Read the model definition and answer for the solid it produces. Units are mm, in the model's axes. Face numbers are marked on the shaded views. Give positions to 0.01 mm unless a question says otherwise; leave off trailing zeros. Loops run counter-clockwise (first coordinate to the right, second up) from the corner with the lowest first, then second, coordinate; pieces in that order, holes last. Notation, with made-up numbers: (75.25, -5) -> (121.25, -5) arc R26 cw to (121.25, 13) -> close; hole circle Ø1 at (-13.75, -5.75). An arc over 180 degrees is marked (long way). Answer as CSV lines item,"result". Start each with the question number.
```python
from build123d import *

# Parameters (mm, degrees)
SKETCH1_R           = 2.5
SKETCH1_R_2         = 4.9
BOSS_EXTRUDE1_DEPTH = 2


with BuildPart() as part:
    # Sketch1 → Boss-Extrude1 (new body)
    with BuildSketch(Plane.XY):
        with BuildLine():
            Line((-15, 8), (-39.191835885, 8))
            ThreePointArc((-39.191835885, 8), (0, 40), (39.191835885, 8))
            Line((39.191835885, 8), (15, 8))
            Line((15, 8), (15, -8))
            Line((15, -8), (39.191835885, -8))
            ThreePointArc((39.191835885, -8), (0, -40), (-39.191835885, -8))
            Line((-39.191835885, -8), (-15, -8))
            Line((-15, -8), (-15, 8))
        make_face()
        with Locations((0, 19.908720325)):
            Circle(SKETCH1_R, mode=Mode.SUBTRACT)
        with Locations((0, -20.091279675)):
            Circle(SKETCH1_R, mode=Mode.SUBTRACT)
        Circle(SKETCH1_R_2, mode=Mode.SUBTRACT)
    extrude(amount=BOSS_EXTRUDE1_DEPTH)


solid = part.part
```
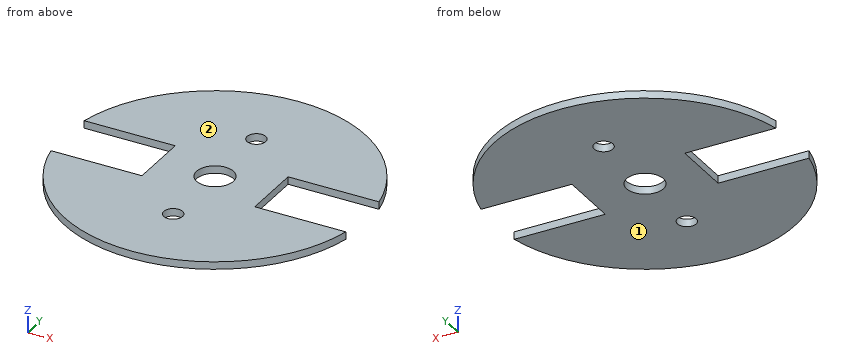
(1) Find the intervals of material crossed by line 1 along Y through (x, z) = (-1, 0.9); line 2 along X through (y, z) = (-20, 0.95); line 3 along X through (y, z) = (-2.5, 1), in increasing order. Write a range as from..to.
(2) Find section D-D on x = 0. Write down the section's boundary in (y, z), then the cut area to 3 significant figures.
(3) Find section C-C on z = 0.9. Write down the section's boundary in (x, y).
(4) Find section B-B on x = 25. Write down the section's boundary in (y, z).
(5) Each of these flat-tipped pins is pushed along its axis until it touches: P1, Ø0.6, axis at x = -28, z = 1, coming from the +Y side; P2, Ø0.6, axis at x = 22.5, z = 1, coming from the +Y side; P3, Ø1, axis at x = -29, z = 1.5, coming from the -Y side. Where does it stop, or does it pass through?
(6) Find section A-A on y = 0. Write down the section's boundary in (x, z), then the cut area to 3 significant figures.
(7) The mould has two halves that part along Z. Classify the marked faces 1 and 2: pulls with the +Z half, pulls with the -Z half, needs draft (parallel to the pull), parting line crosses it, or undercut.
Answer block:
1,line 1,"y = -39.99..-22.38, -17.8..-4.8, 4.8..17.62, 22.2..39.99"
1,line 2,"x = -34.64..-2.5, 2.5..34.64"
1,line 3,"x = -15..-4.21, 4.21..15"
2,outline,"(-40, 0) -> (-22.59, 0) -> (-22.59, 2) -> (-40, 2) -> close; (-17.59, 0) -> (-4.9, 0) -> (-4.9, 2) -> (-17.59, 2) -> close; (4.9, 0) -> (17.41, 0) -> (17.41, 2) -> (4.9, 2) -> close; (22.41, 0) -> (40, 0) -> (40, 2) -> (22.41, 2) -> close"
2,area,"120 mm2"
3,outline,"(-39.19, -8) arc R40 ccw to (39.19, -8) -> (15, -8) -> (15, 8) -> (39.19, 8) arc R40 ccw to (-39.19, 8) -> (-15, 8) -> (-15, -8) -> close; hole circle Ø9.8 at (0, 0); hole circle Ø5 at (0, -20.09); hole circle Ø5 at (0, 19.91)"
4,outline,"(-31.22, 0) -> (-8, 0) -> (-8, 2) -> (-31.22, 2) -> close; (8, 0) -> (31.22, 0) -> (31.22, 2) -> (8, 2) -> close"
5,P1,"stops at y = 28.86"
5,P2,"stops at y = 33.27"
5,P3,"stops at y = -28.07"
6,outline,"(-15, 0) -> (-4.9, 0) -> (-4.9, 2) -> (-15, 2) -> close; (4.9, 0) -> (15, 0) -> (15, 2) -> (4.9, 2) -> close"
6,area,"40.4 mm2"
7,face 1,"pulls with the -Z half"
7,face 2,"pulls with the +Z half"
